Could you check a few things on this model? Use its own coordinates, in mm. A direction names the side the tool comes from. Coordinates: 2 decimals unless noted, no trailing zeros. Write each loop counter-clockwise with the first axis right and the second up, starting at its lowest first coordinate (ties: lowest second). Pieces come first, ordered by that corner, then holes. Notation, with made-up numbers: M 63,60.5 L 113,60.5 A21 cw 113,65.5 Z; hole C -22.75,62.25 d8. An arc over 180 degrees is marked long. Write item = value, one per line.
```python
from build123d import *

# Parameters (mm, degrees)
SKETCH1_W                                           = 115
SKETCH1_H                                           = 85
SKETCH1_R                                           = 8
SKETCH1_W_2                                         = 45.5
SKETCH1_H_2                                         = 22.5
SKETCH1_W_3                                         = 46
BOSS_EXTRUDE1_DEPTH                                 = 5
CSK_FOR_M3_FLAT_COUNTERSUNK_HEAD_SCREW1_D           = 3.4
CSK_FOR_M3_FLAT_COUNTERSUNK_HEAD_SCREW1_CSINK_D     = 6.3
CSK_FOR_M3_FLAT_COUNTERSUNK_HEAD_SCREW1_CSINK_ANGLE = 90


with BuildPart() as part:
    # Sketch1 → Boss-Extrude1 (new body)
    with BuildSketch(Plane(origin=(0, 0, 0), x_dir=(1, 0, 0), z_dir=(0, 1, 0))):
        with Locations((57.5, 42.5)):
            Rectangle(SKETCH1_W, SKETCH1_H)
        with Locations(Location((57.5, 69, 0), (0, 0, 270))):
            Circle(SKETCH1_R, mode=Mode.SUBTRACT)
        with Locations((31.25, 41.25)):
            Rectangle(SKETCH1_W_2, SKETCH1_H_2, mode=Mode.SUBTRACT)
        with Locations((84, 41.25)):
            Rectangle(SKETCH1_W_3, SKETCH1_H_2, mode=Mode.SUBTRACT)
    extrude(amount=-BOSS_EXTRUDE1_DEPTH)

    # CSK for M3 Flat Countersunk Head Screw1 (through all)
    with Locations(Plane(origin=(0, 0, 0), x_dir=(1, 0, 0), z_dir=(0, 1, 0))):
        with Locations((2.5, 65), (2.5, 20), (112.5, 65), (112.5, 20)):
            CounterSinkHole(CSK_FOR_M3_FLAT_COUNTERSUNK_HEAD_SCREW1_D / 2, CSK_FOR_M3_FLAT_COUNTERSUNK_HEAD_SCREW1_CSINK_D / 2, counter_sink_angle=CSK_FOR_M3_FLAT_COUNTERSUNK_HEAD_SCREW1_CSINK_ANGLE)


solid = part.part
```
Item 1: For faces 4 (the face through (115, -2, -42)), 5 (the face through (84, -2, -30)), which set-ups out of +Z, -Z, +X, -X, +Y, -Y let a thin tool reach every point of the face, with its end or its side?
Numbers:
face_4 = +Z, -Z, +X, +Y, -Y
face_5 = +Y, -Y
Item 2: If we mould it in two halves opening along X, with no side actions, what happens to faces 1 (the face through (57, -2, -85)), 2 (the face through (0, -2, -42)), 3 (the face through (114.2, -3.25, -65.07))? For each: pulls with the +X half, pulls with the -X half, needs draft (parallel to the pull), parting line crosses it, or undercut.
Numbers:
face_1 = needs draft
face_2 = pulls with the -X half
face_3 = undercut
Item 3: Imagine slicing it at C-C (y = -2.4). Write out the boundary of the cut face in (x, z).
Numbers:
outline = M 0,-85 L 115,-85 L 115,0 L 0,0 Z; hole C 2.5,-65 d3.4; hole C 2.5,-20 d3.4; hole M 8.5,-52.5 L 54,-52.5 L 54,-30 L 8.5,-30 Z; hole C 57.5,-69 d16; hole M 61,-52.5 L 107,-52.5 L 107,-30 L 61,-30 Z; hole C 112.5,-65 d3.4; hole C 112.5,-20 d3.4
Item 4: If I drill on line 1 along X through (y, z) = (-0.5, -34); line 2 along X through (y, z) = (-3.35, -20); line 3 along Z through (x, y) = (2.5, -2.45), over which ranges is the centre line in solid material (lowest first)?
Numbers:
line_1 = 0 to 8.5, 54 to 61, 107 to 115
line_2 = 0 to 0.8, 4.2 to 110.8, 114.2 to 115
line_3 = -85 to -66.7, -63.3 to -21.7, -18.3 to 0
Item 5: I'm going to push a flat-ended pin straight in: P1, Ø4.5, axis at x = 112.5, z = -65, coming from the +Y side. Where does the tip first touch, or does it pass through?
Numbers:
P1 = -0.9
Item 6: Imagine slicing it at A-A (x = 2.5). Write out the boundary of the cut face in (y, z), and give its area (3 significant figures).
Numbers:
outline = M -5,-85 L 0,-85 L 0,-68.15 L -1.45,-66.7 L -5,-66.7 Z; M -5,-63.3 L -1.45,-63.3 L 0,-61.85 L 0,-23.15 L -1.45,-21.7 L -5,-21.7 Z; M -5,-18.3 L -1.45,-18.3 L 0,-16.85 L 0,0 L -5,0 Z
area = 387 mm²
Item 7: Imagine slicing it at B-B (z = -45). Write out the boundary of the cut face in (x, y).
Numbers:
outline = M 0,-5 L 8.5,-5 L 8.5,0 L 0,0 Z; M 54,-5 L 61,-5 L 61,0 L 54,0 Z; M 107,-5 L 115,-5 L 115,0 L 107,0 Z
Item 8: Imagine slicing it at D-D (x = 57.5). Write out the boundary of the cut face in (y, z).
Numbers:
outline = M -5,-85 L 0,-85 L 0,-77 L -5,-77 Z; M -5,-61 L 0,-61 L 0,0 L -5,0 Z
